```python
from build123d import *

# Parameters (mm, degrees)
SKETCH_1_W      = 55
SKETCH_1_H      = 30
SKETCH_1_R      = 1.5
EXTRUDE_1_DEPTH = 3.5
SKETCH_2_R      = 1.592723526
EXTRUDE_2_DEPTH = 3.5


with BuildPart() as part:
    # 草图1 → 凸台-拉伸1 (new body)
    with BuildSketch(Plane.XY):
        Rectangle(SKETCH_1_W, SKETCH_1_H)
        with Locations((15.634746474, 8.528043531)):
            Circle(SKETCH_1_R, mode=Mode.SUBTRACT)
        with Locations(Location((-15.634746474, 8.528043531, 0), (0, 0, 180))):
            Circle(SKETCH_1_R, mode=Mode.SUBTRACT)
        with Locations(Location((15.634746474, -8.528043531, 0), (0, 0, 180))):
            Circle(SKETCH_1_R, mode=Mode.SUBTRACT)
        with Locations((-15.634746474, -8.528043531)):
            Circle(SKETCH_1_R, mode=Mode.SUBTRACT)
    extrude(amount=EXTRUDE_1_DEPTH)

    # 草图2 → 凸台-拉伸2 (add)
    with BuildSketch(Plane(origin=(27.5, 0, 0), x_dir=(0, 0, -1), z_dir=(1, 0, 0))):
        with BuildLine():
            Line((0, 15), (0, -15))
            Line((0, -15), (21, -15))
            ThreePointArc((21, -15), (36.119015722, 0.838004237), (19.419767517, 15))
            Line((19.419767517, 15), (0, 15))
        make_face()
        with Locations((20, 0)):
            Circle(SKETCH_2_R, mode=Mode.SUBTRACT)
        with Locations(Location((30, 0, 0), (0, 0, 180))):
            Circle(SKETCH_2_R, mode=Mode.SUBTRACT)
    extrude_2 = extrude(amount=-EXTRUDE_2_DEPTH)

    # 镜向1: 凸台-拉伸2 across plane
    add(extrude_2.mirror(Plane(origin=(0, 0, 0), x_dir=(0, 0, 1), z_dir=(1, 0, 0))))


solid = part.part
```
Geometry: final body of the model. Coordinates: model frame, mm. A direction names the side the tool comes from. Round coordinates to 2 decimals unless told otherwise and drop trailing zeros. Write each loop counter-clockwise with the first axis right and the second up, starting at its lowest first coordinate (ties: lowest second). Pieces come first, ordered by that corner, then holes. Notation, with made-up numbers: (66.5, 50.5) -> (109.5, 50.5) arc R33 ccw to (109.5, 80.5) -> close; hole circle Ø4 at (-17.5, 88). An arc over 180 degrees is marked (long way). Return JSON: item names as keys, results as strings.
Q1. First-contact query: pin 1 Ø4 at (y, z) = (0, -20) entering from -X; pin 2 Ø4 at (x, y) = (15.63, -8.53) entering from -Z. Flat tips, straight axial feed; report the tip coordinate or a pass-through.
From the geometry:
{"pin 1": "x = -27.5", "pin 2": "z = 0"}
Q2. Ray query, line 1 (X direction, y = -6, z = -23.5); line 2 (Z direction, x = -16.5, y = 0); line 3 (Y direction, x = 26, z = -30). Return the intervals inside material, ascending.
From the geometry:
{"line 1": "-27.5 to -24, 24 to 27.5", "line 2": "0 to 3.5", "line 3": "-12.08 to -1.59, 1.59 to 12.17"}
Q3. Section D-D on y = 6. Return the cut outline in (x, z), and give its area (3 significant figures).
From the geometry:
{"outline": "(-27.5, -34.91) -> (-24, -34.91) -> (-24, 0) -> (24, 0) -> (24, -34.91) -> (27.5, -34.91) -> (27.5, 3.5) -> (-27.5, 3.5) -> close", "area": "437 mm2"}
Q4. Section B-B on y = 0. Return the cut outline in (x, z), and give its area (3 significant figures).
From the geometry:
{"outline": "(-27.5, -36.14) -> (-24, -36.14) -> (-24, -31.59) -> (-27.5, -31.59) -> close; (-27.5, -28.41) -> (-24, -28.41) -> (-24, -21.59) -> (-27.5, -21.59) -> close; (-27.5, -18.41) -> (-24, -18.41) -> (-24, 0) -> (24, 0) -> (24, -18.41) -> (27.5, -18.41) -> (27.5, 3.5) -> (-27.5, 3.5) -> close; (24, -36.14) -> (27.5, -36.14) -> (27.5, -31.59) -> (24, -31.59) -> close; (24, -28.41) -> (27.5, -28.41) -> (27.5, -21.59) -> (24, -21.59) -> close", "area": "401 mm2"}
Q5. Section A-A on z = -17. Return the cut outline in (x, y).
From the geometry:
{"outline": "(-27.5, -15) -> (-24, -15) -> (-24, 15) -> (-27.5, 15) -> close; (24, -15) -> (27.5, -15) -> (27.5, 15) -> (24, 15) -> close"}
Q6. Set-up query: faces 4 (the flat face through (1.9, -15, 0.4)), 5 (the flat face through (-0.1, 15, 0.5)), 6 (the flat face through (0, 0, 0)). Return all of +Z, -Z, +X, -X, +Y, -Y with unobstructed straight access to the full face (end or side cutting, diameter ignored); none if empty.
From the geometry:
{"face 4": "+Z, -Z, +X, -X, -Y", "face 5": "+Z, +X, -X, +Y", "face 6": "-Z, +Y, -Y"}
Q7. Section C-C on z = -30. Return the cut outline in (x, y), and give its area (3 significant figures).
From the geometry:
{"outline": "(-27.5, -12.08) -> (-24, -12.08) -> (-24, -1.59) -> (-27.5, -1.59) -> close; (-27.5, 1.59) -> (-24, 1.59) -> (-24, 12.17) -> (-27.5, 12.17) -> close; (24, -12.08) -> (27.5, -12.08) -> (27.5, -1.59) -> (24, -1.59) -> close; (24, 1.59) -> (27.5, 1.59) -> (27.5, 12.17) -> (24, 12.17) -> close", "area": "147 mm2"}
Q8. Mould query, pull axis X, two halves, no side actions, for faces 1 (the cylindrical face through (25.77, 0.07, -18.41)), 2 (the cylindrical face through (17.065, 8.979, 1.726)), 3 (the flat face through (27.5, 0, -16)). Classes: +X half, -X half, draft (parallel to the pull), parting line (faces both ways), or undercut.
From the geometry:
{"face 1": "draft", "face 2": "undercut", "face 3": "+X half"}
